For this review, take the finished solid that the model builds, in its own axes (mm). Face numbers are marked on the shaded views. A direction names the side the tool comes from. Coordinates: 2 decimals unless noted, no trailing zeros. Loops run counter-clockwise (first coordinate to the right, second up) from the corner with the lowest first, then second, coordinate; pieces in that order, holes last. Notation, with made-up numbers: (65, 64.5) - (114, 64.5) arc R14 cw to (114, 89.5) - close; hole circle Ø4 at (-13, 22). An arc over 180 degrees is marked (long way). Use one line per item in the form item = value. Start each with the question number.
1. Draft analysis for pull direction Z (two halves, no side actions). For the marked faces 1, 2 and 3, state which applies: +Z half, -Z half, draft (parallel to the pull), parting line (faces both ways), or undercut.
2. Add section A-A on z = 0. Give the boundary of the cut face in (x, y) (3 decimals).
3. Add section B-B on y = 22.5. Give the boundary of the cut face in (x, z), and give its area (3 significant figures).
4. For pin 1 Ø2 at (x, z) = (10.5, 9) entering from -Y; pin 2 Ø12 at (y, z) = (40, 3) entering from +X; pin 3 Ø10 at (y, z) = (5, 2.5) entering from -X; pin 4 Ø6 at (x, z) = (23.5, 9.5) entering from +Y, all flat-tipped, find the tip position at first contact; note any pin that passes through.
5. To check wall thickness, follow probe 1 along X at (y, z) = (45, -18.35); probe 2 along Y at (x, z) = (10, -16.3); probe 3 along Z at (x, y) = (0, 59) (3 decimals). State the ranges of each line that lie inside material, in increasing order.
6. Add section C-C on x = 7. Give the boundary of the cut face in (y, z), and give its area (3 significant figures).
7. Add section D-D on z = -18. Give the boundary of the cut face in (x, y), and give its area (3 significant figures).
8. Machinability: for the marked faces 4, 5, 6, 7 and 8, which of the approach directions +Z, -Z, +X, -X, +Y, -Y give a long, thin tool a straight path to every point of the face, cutting with its end or side? Answer none if there is none.
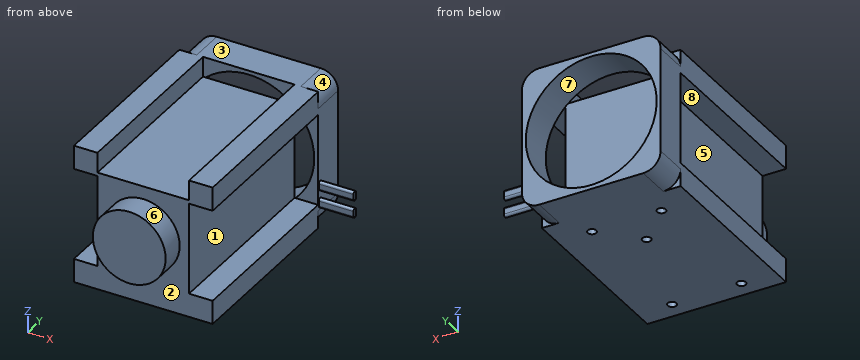
```python
from build123d import *

# Parameters (mm, degrees)
SKETCH1_W                 = 40
SKETCH1_H                 = 40
BOSS_EXTRUDE1_DEPTH       = 62.75
SKETCH2_R                 = 18.875
CUT_EXTRUDE1_DEPTH        = 10
SKETCH4_R                 = 10.5
BOSS_EXTRUDE2_DEPTH       = 7
SKETCH5_W                 = 26.4
SKETCH5_H                 = 5.8
SKETCH5_W_2               = 6.8
SKETCH5_H_2               = 26.4
CUT_EXTRUDE2_DEPTH        = 52.75
M3X0_5_TAPPED_HOLE1_D     = 2.5
M3X0_5_TAPPED_HOLE1_DEPTH = 5
M3X0_5_TAPPED_HOLE1_TIP   = 0.751075774
BOSS_EXTRUDE3_DEPTH       = 10


with BuildPart() as part:
    # Sketch1 → Boss-Extrude1 (new body)
    with BuildSketch(Plane(origin=(0, 0, 0), x_dir=(1, 0, 0), z_dir=(0, 1, 0))):
        Rectangle(SKETCH1_W, SKETCH1_H)
    extrude(amount=BOSS_EXTRUDE1_DEPTH)

    # Sketch2 → Cut-Extrude1 (cut)
    with BuildSketch(Plane(origin=(0, 62.75, 0), x_dir=(1, 0, 0), z_dir=(0, 1, 0))):
        Circle(SKETCH2_R)
        with BuildLine():
            ThreePointArc((-15, -20), (-18.535533906, -18.535533906), (-20, -15))
            Line((-20, -15), (-20, -20))
            Line((-20, -20), (-15, -20))
        make_face()
        with BuildLine():
            ThreePointArc((20, -15), (18.535533906, -18.535533906), (15, -20))
            Line((15, -20), (20, -20))
            Line((20, -20), (20, -15))
        make_face()
        with BuildLine():
            Line((20, 20), (15, 20))
            ThreePointArc((15, 20), (18.535533906, 18.535533906), (20, 15))
            Line((20, 15), (20, 20))
        make_face()
        with BuildLine():
            Line((-15, 20), (-20, 20))
            Line((-20, 20), (-20, 15))
            ThreePointArc((-20, 15), (-18.535533906, 18.535533906), (-15, 20))
        make_face()
    extrude(amount=-CUT_EXTRUDE1_DEPTH, mode=Mode.SUBTRACT)

    # Sketch4 → Boss-Extrude2 (add)
    with BuildSketch(Plane.XZ):
        Circle(SKETCH4_R)
    extrude(amount=BOSS_EXTRUDE2_DEPTH)

    # Sketch5 → Cut-Extrude2 (cut)
    with BuildSketch(Plane.XZ):
        with Locations((0, 17.1)):
            Rectangle(SKETCH5_W, SKETCH5_H)
        with Locations((16.6, 0)):
            Rectangle(SKETCH5_W_2, SKETCH5_H_2)
        with Locations((-16.6, 0)):
            Rectangle(SKETCH5_W_2, SKETCH5_H_2)
    extrude(amount=-CUT_EXTRUDE2_DEPTH, mode=Mode.SUBTRACT)

    # M3x0.5 Tapped Hole1
    with Locations(Plane(origin=(0, 0, -20), x_dir=(-1, 0, 0), z_dir=(0, 0, -1))):
        with Locations((-10, 45), (10, 45), (10, 5), (-10, 5), (0, 35)):
            Hole(M3X0_5_TAPPED_HOLE1_D / 2, depth=M3X0_5_TAPPED_HOLE1_DEPTH)
            with Locations((0, 0, -(M3X0_5_TAPPED_HOLE1_DEPTH + M3X0_5_TAPPED_HOLE1_TIP / 2))):  # 118° drill point
                Cone(0, M3X0_5_TAPPED_HOLE1_D / 2, M3X0_5_TAPPED_HOLE1_TIP, mode=Mode.SUBTRACT)

    # Sketch9 → Boss-Extrude3 (add)
    with BuildSketch(Plane(origin=(20, 0, 0), x_dir=(0, 0, -1), z_dir=(1, 0, 0))):
        with BuildLine():
            Line((7.275, 54.4), (8.725, 54.4))
            ThreePointArc((8.725, 54.4), (9.375, 53.75), (8.725, 53.1))
            Line((8.725, 53.1), (7.275, 53.1))
            ThreePointArc((7.275, 53.1), (6.625, 53.75), (7.275, 54.4))
        make_face()
        with BuildLine():
            Line((12.275, 54.4), (13.725, 54.4))
            ThreePointArc((13.725, 54.4), (14.375, 53.75), (13.725, 53.1))
            Line((13.725, 53.1), (12.275, 53.1))
            ThreePointArc((12.275, 53.1), (11.625, 53.75), (12.275, 54.4))
        make_face()
    extrude(amount=BOSS_EXTRUDE3_DEPTH)


solid = part.part
```
Conclusion:
q1.face_1 = undercut
q1.face_2 = draft
q1.face_3 = +Z half
q2.outline = (-20, 52.75) - (-18.875, 52.75) - (-18.875, 62.75) - (-20, 62.75) - close; (-13.2, 0) - (-10.5, 0) - (-10.5, -7) - (10.5, -7) - (10.5, 0) - (13.2, 0) - (13.2, 52.75) - (-13.2, 52.75) - close; (18.875, 52.75) - (20, 52.75) - (20, 62.75) - (18.875, 62.75) - close
q3.outline = (-20, -20) - (20, -20) - (20, -13.2) - (13.2, -13.2) - (13.2, 13.2) - (20, 13.2) - (20, 20) - (13.2, 20) - (13.2, 14.2) - (-13.2, 14.2) - (-13.2, 20) - (-20, 20) - (-20, 13.2) - (-13.2, 13.2) - (-13.2, -13.2) - (-20, -13.2) - close
q3.area = 1,090 mm^2
q4.pin_1 = 0
q4.pin_2 = 13.2
q4.pin_3 = -13.2
q4.pin_4 = through
q5.probe_1 = -20 to -11.25, -8.75 to 8.75, 11.25 to 20
q5.probe_2 = 0 to 3.75, 6.25 to 43.75, 46.25 to 62.75
q5.probe_3 = -20 to -18.875, 18.875 to 20
q6.outline = (-7, -7.83) - (0, -7.83) - (0, -20) - (62.75, -20) - (62.75, -17.53) - (52.75, -17.53) - (52.75, 14.2) - (0, 14.2) - (0, 7.83) - (-7, 7.83) - close; (52.75, 17.53) - (62.75, 17.53) - (62.75, 20) - (52.75, 20) - close
q6.area = 1,960 mm^2
q7.outline = (-20, 0) - (20, 0) - (20, 52.75) - (19, 52.75) - (19, 62.75) - (5.68, 62.75) - (5.68, 52.75) - (-5.68, 52.75) - (-5.68, 62.75) - (-19, 62.75) - (-19, 52.75) - (-20, 52.75) - close; hole circle Ø2.5 at (-10, 5); hole circle Ø2.5 at (-10, 45); hole circle Ø2.5 at (0, 35); hole circle Ø2.5 at (10, 5); hole circle Ø2.5 at (10, 45)
q7.area = 2,350 mm^2
q8.face_4 = +Z, +X, +Y
q8.face_5 = -X, +Y, -Y
q8.face_6 = -Y
q8.face_7 = +Y
q8.face_8 = -X, -Y
